```python
from build123d import *

# Parameters (mm, degrees)
BOSS_EXTRUDE1_DEPTH = 9.525
SKETCH2_R           = 3.96875
BOSS_EXTRUDE2_DEPTH = 6.35


with BuildPart() as part:
    # Sketch1 → Boss-Extrude1 (new, symmetric)
    with BuildSketch(Plane.XY):
        with BuildLine():
            Line((-10.066701328, 1.984375), (-10.066701328, -1.984375))
            Line((-10.066701328, -1.984375), (-7.685451328, -1.984375))
            ThreePointArc((-7.685451328, -1.984375), (-6.874076643, -3.96875), (-5.561244824, -5.663608589))
            Line((-5.561244824, -5.663608589), (-6.751869824, -7.725831582))
            Line((-6.751869824, -7.725831582), (-3.314831503, -9.710206582))
            Line((-3.314831503, -9.710206582), (-2.124206503, -7.647983589))
            ThreePointArc((-2.124206503, -7.647983589), (0, -7.9375), (2.124206503, -7.647983589))
            Line((2.124206503, -7.647983589), (3.314831503, -9.710206582))
            Line((3.314831503, -9.710206582), (6.751869824, -7.725831582))
            Line((6.751869824, -7.725831582), (5.561244824, -5.663608589))
            ThreePointArc((5.561244824, -5.663608589), (6.874076643, -3.96875), (7.685451328, -1.984375))
            Line((7.685451328, -1.984375), (10.066701328, -1.984375))
            Line((10.066701328, -1.984375), (10.066701328, 1.984375))
            Line((10.066701328, 1.984375), (7.685451328, 1.984375))
            ThreePointArc((7.685451328, 1.984375), (6.874076643, 3.96875), (5.561244824, 5.663608589))
            Line((5.561244824, 5.663608589), (6.751869824, 7.725831582))
            Line((6.751869824, 7.725831582), (3.314831503, 9.710206582))
            Line((3.314831503, 9.710206582), (2.124206503, 7.647983589))
            ThreePointArc((2.124206503, 7.647983589), (0, 7.9375), (-2.124206503, 7.647983589))
            Line((-2.124206503, 7.647983589), (-3.314831503, 9.710206582))
            Line((-3.314831503, 9.710206582), (-6.751869824, 7.725831582))
            Line((-6.751869824, 7.725831582), (-5.561244824, 5.663608589))
            ThreePointArc((-5.561244824, 5.663608589), (-6.874076643, 3.96875), (-7.685451328, 1.984375))
            Line((-7.685451328, 1.984375), (-10.066701328, 1.984375))
        make_face()
    extrude(amount=BOSS_EXTRUDE1_DEPTH, both=True)

    # Sketch2 → Boss-Extrude2 (add)
    with BuildSketch(Plane.XY.offset(9.525)):
        Circle(SKETCH2_R)
    extrude(amount=BOSS_EXTRUDE2_DEPTH)


solid = part.part
```
Can you work these out from the model? Positions are in its coordinate system, mm. A direction names the side the tool comes from. Give positions to 0.01 mm unless a question says otherwise; leave off trailing zeros. Write each loop counter-clockwise with the first axis right and the second up, starting at its lowest first coordinate (ties: lowest second). Pieces come first, ordered by that corner, then holes. Notation, with made-up numbers: (-27.5, 30) - (-23.5, 30) arc R35 ccw to (-23.5, 66) - close; hole circle Ø11 at (-9.5, 19). An arc over 180 degrees is marked (long way). Write item = value, one per line. Start each with the question number.
1. Imagine slicing it at B-B (x = 6.25). Please give me the cut outline in (y, z) (3 decimals).
2. For pin 1 (1.9 mm diameter, centred on x = -9, z = -3, fed in from -Y); pin 2 (6 mm diameter, centred on x = -7.5, z = 9, fed in from -Y); pin 3 (10 mm diameter, centred on x = 7.5, z = 4, fed in from +Y), each with a flat end and sliding along its axis, tell me the tip position at first contact or that it passes through.
3. Thinking about a two-plate mould opening in X: for faces 5 (the face through (-2.728, -8.694, 0.133)), 6 (the face through (6.15, 6.68, 0.13)), 7 (the face through (-0.86, -3.874, 12.656)), which applies, released by +X, released by -X, zero draft, split by the parting line, or undercut?
4. Imagine slicing it at C-C (z = -5.5). Please give me the cut outline in (x, y) (1 decimal), and give its area (3 significant figures).
5. On a 3-axis mill with a long thin cutter (end or side, diameter ignored), from which of +Z, -Z, +X, -X, +Y, -Y can I reach the whole of each face in a straight line? I mean faces 1 (the face through (-6.165, 6.709, 0.133)), 2 (the face through (-9, 1.984, 0)), 3 (the face through (9, -1.984, 0)), 4 (the face through (4.3, 0.1, 9.525)). Say none if no direction works.
6. Please list where these lines run through material, in increasing order: line 1 (Z direction, x = -3, y = 5.75) (3 decimals); line 2 (Y direction, x = -6.5, z = 2.25); line 3 (Y direction, x = 0, z = -4.5).
7. Imagine slicing it at A-A (y = -8.25). Please give me the cut outline in (x, z) (3 decimals), and give its area (3 significant figures).
8. Imagine slicing it at D-D (x = 0). Please give me the cut outline in (y, z) (1 decimal).
Worked answers:
q1.outline = (-8.016, -9.525) - (-6.857, -9.525) - (-6.857, 9.525) - (-8.016, 9.525) - close; (-4.893, -9.525) - (4.893, -9.525) - (4.893, 9.525) - (-4.893, 9.525) - close; (6.857, -9.525) - (8.016, -9.525) - (8.016, 9.525) - (6.857, 9.525) - close
q2.pin_1 = -1.98
q2.pin_2 = -9.03
q2.pin_3 = 9.71
q3.face_5 = undercut
q3.face_6 = released by +X
q3.face_7 = split by the parting line
q4.outline = (-10.1, -2) - (-7.7, -2) arc R7.9 ccw to (-5.6, -5.7) - (-6.8, -7.7) - (-3.3, -9.7) - (-2.1, -7.6) arc R7.9 ccw to (2.1, -7.6) - (3.3, -9.7) - (6.8, -7.7) - (5.6, -5.7) arc R7.9 ccw to (7.7, -2) - (10.1, -2) - (10.1, 2) - (7.7, 2) arc R7.9 ccw to (5.6, 5.7) - (6.8, 7.7) - (3.3, 9.7) - (2.1, 7.6) arc R7.9 ccw to (-2.1, 7.6) - (-3.3, 9.7) - (-6.8, 7.7) - (-5.6, 5.7) arc R7.9 ccw to (-7.7, 2) - (-10.1, 2) - close
q4.area = 251 mm2
q5.face_1 = +Z, -Z, -X
q5.face_2 = +Z, -Z, -X, +Y
q5.face_3 = +Z, -Z, +X, -Y
q5.face_4 = +Z
q6.line_1 = -9.525 to 9.525
q6.line_2 = -7.87 to -7.29, -4.56 to 4.56, 7.29 to 7.87
q6.line_3 = -7.94 to 7.94
q7.outline = (-5.844, -9.525) - (-2.472, -9.525) - (-2.472, 9.525) - (-5.844, 9.525) - close; (2.472, -9.525) - (5.844, -9.525) - (5.844, 9.525) - (2.472, 9.525) - close
q7.area = 128 mm2
q8.outline = (-7.9, -9.5) - (7.9, -9.5) - (7.9, 9.5) - (4, 9.5) - (4, 15.9) - (-4, 15.9) - (-4, 9.5) - (-7.9, 9.5) - close
